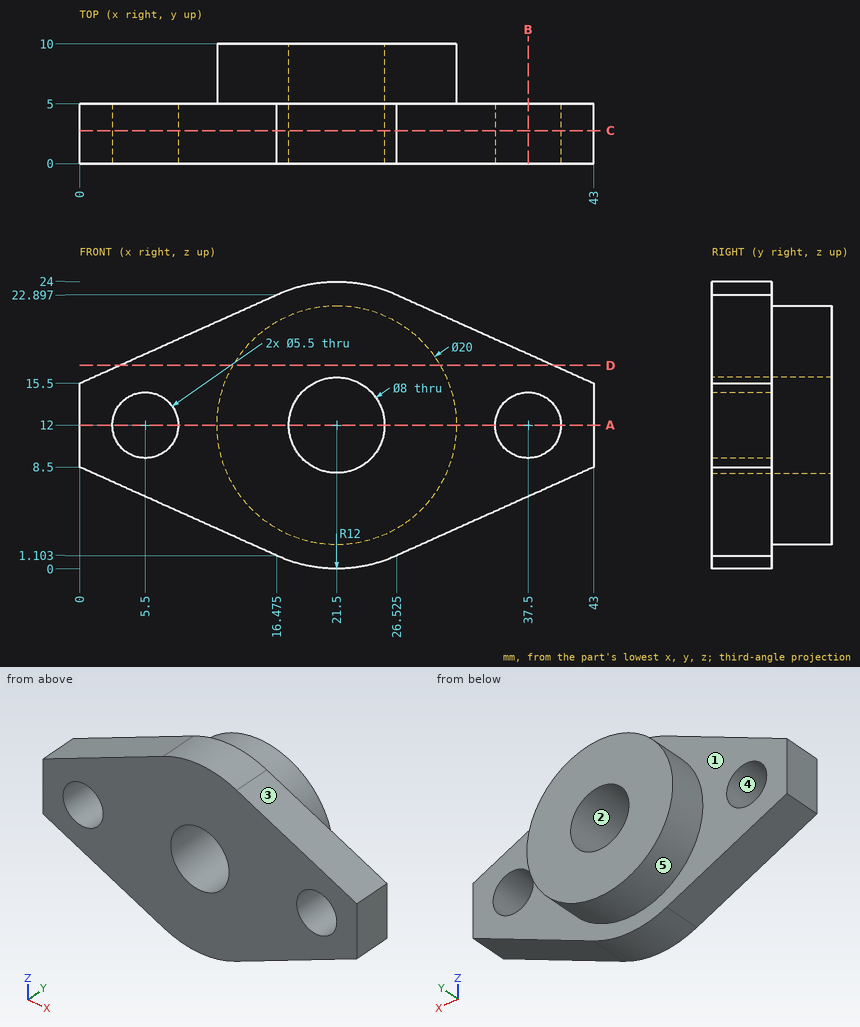
Part print with two shaded views. Sizes in mm from the minimum x, y, z corner. A direction names the side the tool comes from. Give positions to 0.01 mm unless a question says otherwise; leave off trailing zeros. Order: outer loops, then holes, each group sorted by start corner. A loop starts at its lowest first (then second) coordinate and runs counter-clockwise, first axis right, second up.
1) Saw through at D-D, the plane z = 17. Write the cut outline in (x, y), then the cut area to 3 significant figures.
2) 3-axis set-ups, long thin cutter, end or side, ignore diameter. For the marked faces 4 and 5: which of +Z, -Z, +X, -X, +Y, -Y reach the whole face in a straight line?
3) Saw through at B-B, the plane x = 37.5. Write the cut outline in (y, z).
4) Pin check, flat tips, straight feed: pin 1 (6.5 mm diameter, centred on x = 5.5, z = 12, fed in from +Y); pin 2 (2 mm diameter, centred on x = 9.5, y = 2, fed in from -Z) (1 decimal); pin 3 (5 mm diameter, centred on x = 16.5, y = 2.5, fed in from +Z). Stop position of each tip, or through.
5) Mould opens along Z. For the marked faces 1, 2 and 3 say: +Z half, -Z half, draft (parallel to the pull), parting line (faces both ways), or undercut.
6) Saw through at A-A, the plane z = 12. Write the cut outline in (x, y), then the cut area to 3 significant figures.
7) Saw through at C-C, the plane y = 2.75. Count the separate pieces of the cut face and the enclosed holes in it.
8) Wall check: probe 1 along X at (y, z) = (1.7, 12); probe 2 along X at (y, z) = (6.75, 12); probe 3 along Y at (x, z) = (10, 15.25). Give the ranges that are in metal, low to high.
Computed:
1. outline: (3.34, 0) - (39.66, 0) - (39.66, 5) - (30.16, 5) - (30.16, 10) - (12.84, 10) - (12.84, 5) - (3.34, 5) - close
1. area: 268 mm2
2. face 4: +Y, -Y
2. face 5: +Y
3. outline: (0, 6.03) - (5, 6.03) - (5, 9.25) - (0, 9.25) - close; (0, 14.75) - (5, 14.75) - (5, 17.97) - (0, 17.97) - close
4. pin 1: stops at y = 5
4. pin 2: stops at z = 3.8
4. pin 3: stops at z = 23.74
5. face 1: draft
5. face 2: undercut
5. face 3: +Z half
6. outline: (0, 0) - (2.75, 0) - (2.75, 5) - (0, 5) - close; (8.25, 0) - (17.5, 0) - (17.5, 10) - (11.5, 10) - (11.5, 5) - (8.25, 5) - close; (25.5, 0) - (34.75, 0) - (34.75, 5) - (31.5, 5) - (31.5, 10) - (25.5, 10) - close; (40.25, 0) - (43, 0) - (43, 5) - (40.25, 5) - close
6. area: 180 mm2
7. separate pieces: 1
7. enclosed holes: 3
8. probe 1: x = 0 to 2.75, 8.25 to 17.5, 25.5 to 34.75, 40.25 to 43
8. probe 2: x = 11.5 to 17.5, 25.5 to 31.5
8. probe 3: y = 0 to 5
